Could you check a few things on this drawing? It's one solid part, dimensions in mm from its lowest x, y, z. A direction names the side the tool comes from. Coordinates: 2 decimals unless noted, no trailing zeros. Loops run counter-clockwise (first coordinate to the right, second up) from the corner with the lowest first, then second, coordinate; pieces in that order, holes last.
1) Imagine slicing it at D-D on z = 2.75. Please give me the cut outline in (x, y).
2) Thinking about a two-plate mould opening in Y: for the marked faces 1, 2, 3 and 4, which applies, released by +Y, released by -Y, zero draft, split by the parting line, or undercut?
3) Imagine slicing it at C-C on y = 9.5. Please give me the cut outline in (x, z).
4) Will these pins go through, and if not, where does the flat tip stop? P1, Ø4, axis at x = 5, y = 8.5, coming from the -Z side; P2, Ø0.9, axis at x = 0.5, y = 14, coming from the -Z side; P3, Ø3, axis at x = 5, y = 10, coming from the -Z side; P4, Ø0.6, axis at x = 0.5, z = 4, coming from the -Y side.
5) For the marked faces 5, 6, 7 and 8, which set-ups out of +Z, -Z, +X, -X, +Y, -Y let a thin tool reach every point of the face, with its end or its side?
6) Imagine slicing it at A-A on z = 3.5. Please give me the cut outline in (x, y).
7) Imagine slicing it at B-B on x = 4.5. Please give me the cut outline in (y, z).
8) If I drill on line 1 along Y through (x, z) = (3, 1.5); line 2 along X through (y, z) = (3.75, 3.5); line 3 along Z through (x, y) = (0.5, 16.75), over which ranges is the centre line in solid material (lowest first)?
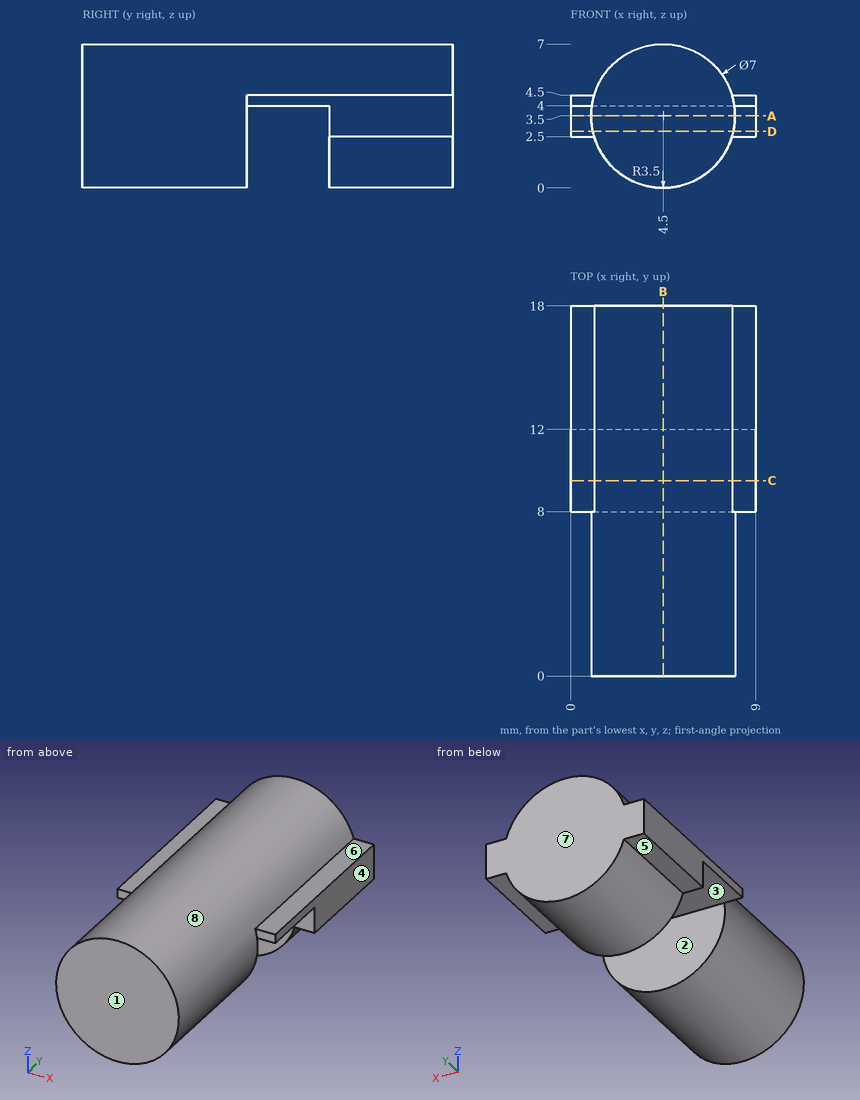
Filled in:
1. outline: (0, 12) - (9, 12) - (9, 18) - (0, 18) - close; (1.08, 0) - (7.92, 0) - (7.92, 8) - (1.08, 8) - close
2. face 1: released by -Y
2. face 2: undercut
2. face 3: undercut
2. face 4: zero draft
3. outline: (0, 4) - (9, 4) - (9, 4.5) - (7.85, 4.5) arc R3.5 ccw to (1.15, 4.5) - (0, 4.5) - close
4. P1: stops at z = 0
4. P2: stops at z = 2.5
4. P3: stops at z = 4
4. P4: stops at y = 8
5. face 5: -Z, -X, +Y, -Y
5. face 6: +Z, +X, +Y, -Y
5. face 7: +Z, -Z, +X, -X, +Y
5. face 8: -Y
6. outline: (0, 12) - (9, 12) - (9, 18) - (0, 18) - close; (1, 0) - (8, 0) - (8, 8) - (1, 8) - close
7. outline: (0, 0) - (8, 0) - (8, 4) - (12, 4) - (12, 0) - (18, 0) - (18, 7) - (0, 7) - close
8. line 1: y = 0 to 8, 12 to 18
8. line 2: x = 1 to 8
8. line 3: z = 2.5 to 4.5
